```python
from build123d import *

# Parameters (mm, degrees)
BOSS_EXTRUDE1_DEPTH                                  = 5
CBORE_FOR_M3_HEX_SOCKET_THIN_HEAD_CAP_SC_D           = 3.6
CBORE_FOR_M3_HEX_SOCKET_THIN_HEAD_CAP_SC_CBORE_D     = 6.5
CBORE_FOR_M3_HEX_SOCKET_THIN_HEAD_CAP_SC_CBORE_DEPTH = 2.4
CBORE_FOR_M3_HEX_SOCKET_THIN_HEAD_CA_2_D             = 3.6
CBORE_FOR_M3_HEX_SOCKET_THIN_HEAD_CA_2_CBORE_D       = 6.5
CBORE_FOR_M3_HEX_SOCKET_THIN_HEAD_CA_2_CBORE_DEPTH   = 2.4
FILLET1_R                                            = 3.175
FILLET2_R                                            = 1.5875


with BuildPart() as part:
    # Sketch1 → Boss-Extrude1 (new, symmetric)
    with BuildSketch(Plane.XY):
        Polygon((0, 0), (20, 0), (20, 5), (5, 5), (5, 20), (0, 20), align=None)
    extrude(amount=BOSS_EXTRUDE1_DEPTH, both=True)

    # CBORE for M3 Hex Socket Thin Head Cap Sc (through all)
    with Locations(Plane(origin=(5, 0, 0), x_dir=(0, 0, -1), z_dir=(1, 0, 0))):
        with Locations((0, 10.475)):
            CounterBoreHole(CBORE_FOR_M3_HEX_SOCKET_THIN_HEAD_CAP_SC_D / 2, CBORE_FOR_M3_HEX_SOCKET_THIN_HEAD_CAP_SC_CBORE_D / 2, CBORE_FOR_M3_HEX_SOCKET_THIN_HEAD_CAP_SC_CBORE_DEPTH)

    # CBORE for M3 Hex Socket Thin Head Ca 2 (through all)
    with Locations(Plane(origin=(0, 5, 0), x_dir=(1, 0, 0), z_dir=(0, 1, 0))):
        with Locations((10.475, 0)):
            CounterBoreHole(CBORE_FOR_M3_HEX_SOCKET_THIN_HEAD_CA_2_D / 2, CBORE_FOR_M3_HEX_SOCKET_THIN_HEAD_CA_2_CBORE_D / 2, CBORE_FOR_M3_HEX_SOCKET_THIN_HEAD_CA_2_CBORE_DEPTH)

    # Fillet1
    fillet1_edges = [part.edges().sort_by_distance(p)[0] for p in [
        (5, 20, 0),
        (20, 5, 0),
    ]]
    fillet(fillet1_edges, radius=FILLET1_R)

    # Fillet2
    fillet2_edges = [part.edges().sort_by_distance(p)[0] for p in [
        (20, 0.9125, 5),
        (5, 10.9125, 5),
        (10.9125, 5, -5),
        (10.9125, 5, 5),
        (0.9125, 20, -5),
        (4.07006403, 19.07006403, -5),
        (19.07006403, 4.07006403, -5),
        (0.9125, 20, 5),
        (4.07006403, 19.07006403, 5),
        (19.07006403, 4.07006403, 5),
        (5, 10.9125, -5),
        (20, 0.9125, -5),
    ]]
    fillet(fillet2_edges, radius=FILLET2_R)


solid = part.part
```
Input: part model. Units: mm. Frame: model coordinates. A direction names the side the tool comes from. Coordinates: 2 decimals unless noted, no trailing zeros. Write each loop counter-clockwise with the first axis right and the second up, starting at its lowest first coordinate (ties: lowest second). Pieces come first, ordered by that corner, then holes.
1) Section D-D on y = 14. Output: boundary loops of the cut face in (x, z) (1 decimal).
2) Pin query (flat end, axial travel): pin 1 Ø1.5 at (x, y) = (13, 4.5) entering from +Z; pin 2 Ø3 at (x, z) = (10.5, -0.5) entering from +Y; pin 3 Ø5 at (y, z) = (9.5, 1) entering from +X. Return the tip coordinate at first contact, or that it passes through.
3) Material intervals for line 1 along Y through (x, z) = (1, 0) (3 decimals); line 2 along X through (y, z) = (13, -3); line 3 along X through (y, z) = (10.5, 2.75), sorted ascending.
4) Set-up query: faces 1 (the cylindrical face through (3.8, 7.3, 0.7)), 2 (the cylindrical face through (10.02, 4.55, 4.52)), 3 (the cylindrical face through (10.02, 4.52, -4.55)), 4 (the cylindrical face through (13.48, 3.82, 1.24)), 5 (the flat face through (5, 13.5, 1.6)). Return all of +Z, -Z, +X, -X, +Y, -Y with unobstructed straight access to the full face (end or side cutting, diameter ignored); none if empty.
5) Mould query, pull axis Z, two halves, no side actions, for faces 6 (the cylindrical face through (1.282, 8.718, -0.39)), 7 (the cylindrical face through (0.9, 19.55, 4.52)), 8 (the flat face through (14, 5, 2)). Classes: pulls with the +Z half, pulls with the -Z half, needs draft (parallel to the pull), parting line crosses it, or undercut.
6) Section B-B on z = 0. Output: boundary loops of the cut face in (x, y) (3 decimals).
Check result:
1. outline: (0, -5) - (3.4, -5) arc R1.6 ccw to (5, -3.4) - (5, 3.4) arc R1.6 ccw to (3.4, 5) - (0, 5) - close
2. pin 1: stops at z = 4.96
2. pin 2: stops at y = 2.6
2. pin 3: stops at x = 5
3. line 1: y = 0 to 8.675, 12.275 to 20
3. line 2: x = 0 to 5
3. line 3: x = 0 to 2.6
4. face 1: +X
4. face 2: +Z, +X, +Y
4. face 3: -Z, +X, +Y
4. face 4: +Y
4. face 5: +Z, -Z, +X, +Y
5. face 6: undercut
5. face 7: pulls with the +Z half
5. face 8: needs draft
6. outline: (0, 0) - (8.675, 0) - (8.675, 2.6) - (7.225, 2.6) - (7.225, 5) - (5, 5) - (5, 7.225) - (2.6, 7.225) - (2.6, 8.675) - (0, 8.675) - close; (0, 12.275) - (2.6, 12.275) - (2.6, 13.725) - (5, 13.725) - (5, 16.825) arc R3.175 ccw to (1.825, 20) - (0, 20) - close; (12.275, 0) - (20, 0) - (20, 1.825) arc R3.175 ccw to (16.825, 5) - (13.725, 5) - (13.725, 2.6) - (12.275, 2.6) - close
